Read the model definition and answer for the solid it produces. Units are mm, in the model's axes. Face numbers are marked on the shaded views. A direction names the side the tool comes from. Coordinates: 2 decimals unless noted, no trailing zeros. Write each loop counter-clockwise with the first axis right and the second up, starting at its lowest first coordinate (ties: lowest second). Pieces come first, ordered by that corner, then holes. Notation, with made-up numbers: (28.5, 61.25) -> (55.5, 61.25) arc R27 cw to (55.5, 97.25) -> close; hole circle Ø1 at (85.25, 43.25). An arc over 180 degrees is marked (long way). One line per item, written item: value. Start each with the question number.
1. For the marked faces 1, 2 and 3, determine the directions among +Z, -Z, +X, -X, +Y, -Y from which every point of the face is accessible in a straight line to the end or side of a thin tool.
2. Given P1, Ø1.9, axis at y = 16, z = -66, coming from the +X side; P2, Ø9, axis at y = 64.5, z = -59, coming from the +X side; P3, Ø3.5, axis at x = 7.5, y = 61, coming from the +Z side, each flat-ended and moving along its own axis, determine where each tip first touches the part or whether it passes through.
3. Find section C-C, the plane y = 55. Write down the section's boundary in (x, z) (3 decimals).
4. Find section D-D, the plane x = 18. Write down the section's boundary in (y, z) (3 decimals).
5. Consider line 1 along X through (y, z) = (46.5, -60); line 2 along X through (y, z) = (23.5, -91); line 3 along Y through (x, z) = (19, -52.5). Determine where each line is inside the solid, lowest interval first.
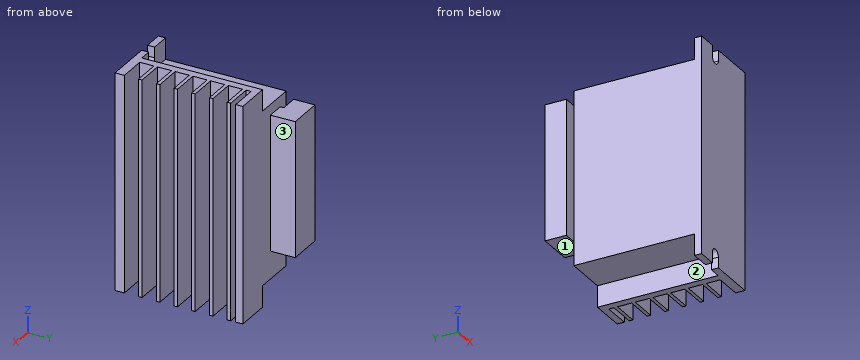
```python
from build123d import *

# Parameters (mm, degrees)
BOSS_EXTRUDE1_DEPTH = 57.15
SKETCH2_W           = 19.05
SKETCH2_H           = 53.975
CUT_EXTRUDE1_DEPTH  = 9.525
SKETCH4_W           = 19.05
SKETCH4_H           = 53.975
CUT_EXTRUDE2_DEPTH  = 9.525
SKETCH5_W           = 12.384603188
SKETCH5_H           = 6.35
SKETCH5_H_2         = 2.244857945
CUT_EXTRUDE3_DEPTH  = 96.52
SKETCH6_W           = 7.9375
SKETCH6_H           = 60.325
BOSS_EXTRUDE2_DEPTH = 1.5875
SKETCH7_W           = 15.875
SKETCH7_H           = 60.325
BOSS_EXTRUDE3_DEPTH = 9.525


with BuildPart() as part:
    # Sketch1 → Boss-Extrude1 (new body)
    with BuildSketch(Plane(origin=(0, 0, 0), x_dir=(1, 0, 0), z_dir=(0, 1, 0))):
        with BuildLine():
            Line((0, 0), (8.73125, 0))
            Line((8.73125, 0), (8.73125, 4.7625))
            ThreePointArc((8.73125, 4.7625), (11.1125, 7.14375), (13.49375, 4.7625))
            Line((13.49375, 4.7625), (13.49375, 0))
            Line((13.49375, 0), (34.925, 0))
            Line((34.925, 0), (34.925, 96.52))
            Line((34.925, 96.52), (13.49375, 96.52))
            Line((13.49375, 96.52), (13.49375, 91.7575))
            ThreePointArc((13.49375, 91.7575), (11.1125, 89.37625), (8.73125, 91.7575))
            Line((8.73125, 91.7575), (8.73125, 96.52))
            Line((8.73125, 96.52), (0, 96.52))
            Line((0, 96.52), (0, 0))
        make_face()
    extrude(amount=BOSS_EXTRUDE1_DEPTH)

    # Sketch2 → Cut-Extrude1 (cut)
    with BuildSketch(Plane.XY):
        with Locations((9.525, 30.1625)):
            Rectangle(SKETCH2_W, SKETCH2_H)
    extrude(amount=-CUT_EXTRUDE1_DEPTH, mode=Mode.SUBTRACT)

    # Sketch4 → Cut-Extrude2 (cut)
    with BuildSketch(Plane(origin=(0, 0, -96.52), x_dir=(-1, 0, 0), z_dir=(0, 0, -1))):
        with Locations((-9.525, 30.1625)):
            Rectangle(SKETCH4_W, SKETCH4_H)
    extrude(amount=-CUT_EXTRUDE2_DEPTH, mode=Mode.SUBTRACT)

    # Sketch5 → Cut-Extrude3 (cut)
    with BuildSketch(Plane(origin=(0, 0, -96.52), x_dir=(-1, 0, 0), z_dir=(0, 0, -1))):
        with Locations((-28.732698406, 7.349133021)):
            Rectangle(SKETCH5_W, SKETCH5_H)
        with Locations((-28.732698406, 15.272834828)):
            Rectangle(SKETCH5_W, SKETCH5_H)
        with Locations((-28.732698406, 23.196536634)):
            Rectangle(SKETCH5_W, SKETCH5_H)
        with Locations((-28.732698406, 31.120238441)):
            Rectangle(SKETCH5_W, SKETCH5_H)
        with Locations((-28.732698406, 39.043940248)):
            Rectangle(SKETCH5_W, SKETCH5_H)
        with Locations((-28.732698406, 46.967642055)):
            Rectangle(SKETCH5_W, SKETCH5_H)
        with Locations((-28.732698406, 52.852571028)):
            Rectangle(SKETCH5_W, SKETCH5_H_2)
    extrude(amount=-CUT_EXTRUDE3_DEPTH, mode=Mode.SUBTRACT)

    # Sketch6 → Boss-Extrude2 (add)
    with BuildSketch(Plane(origin=(0, 57.15, 0), x_dir=(1, 0, 0), z_dir=(0, 1, 0))):
        with Locations((8.73125, 44.448135035)):
            Rectangle(SKETCH6_W, SKETCH6_H)
    extrude(amount=BOSS_EXTRUDE2_DEPTH)

    # Sketch7 → Boss-Extrude3 (add)
    with BuildSketch(Plane(origin=(0, 58.7375, 0), x_dir=(1, 0, 0), z_dir=(0, 1, 0))):
        with Locations((4.7625, 44.448135035)):
            Rectangle(SKETCH7_W, SKETCH7_H)
    extrude(amount=BOSS_EXTRUDE3_DEPTH)


solid = part.part
```
Answer block:
1. face 1: -Z, +X, -X, +Y
1. face 2: -Z, -X, +Y
1. face 3: +Z, -Z, +X, +Y
2. P1: stops at x = 22.54
2. P2: stops at x = 12.7
2. P3: stops at z = -14.29
3. outline: (0, -86.995) -> (19.05, -86.995) -> (19.05, -96.52) -> (34.925, -96.52) -> (34.925, 0) -> (19.05, 0) -> (19.05, -9.525) -> (0, -9.525) -> close
4. outline: (0, -96.52) -> (3.175, -96.52) -> (3.175, -86.995) -> (57.15, -86.995) -> (57.15, -9.525) -> (3.175, -9.525) -> (3.175, 0) -> (0, 0) -> close
5. line 1: x = 0 to 22.54
5. line 2: x = 19.05 to 22.54
5. line 3: y = 0 to 57.15
